from build123d import *

# Parameters (mm, degrees)
SKETCH1_W           = 100
SKETCH1_H           = 100
SKETCH1_R           = 0.75
BOSS_EXTRUDE1_DEPTH = 10
SKETCH2_W           = 110
SKETCH2_H           = 110
SKETCH2_W_2         = 100
SKETCH2_H_2         = 100
BOSS_EXTRUDE3_DEPTH = 5
FILLET2_R           = 2


with BuildPart() as part:
    # Sketch1 → Boss-Extrude1 (new body)
    with BuildSketch(Plane(origin=(0, 0, 0), x_dir=(1, 0, 0), z_dir=(0, 1, 0))):
        Rectangle(SKETCH1_W, SKETCH1_H)
        with Locations(Location((-25, 25, 0), (0, 0, 270))):
            Circle(SKETCH1_R, mode=Mode.SUBTRACT)
        with Locations(Location((25, -25, 0), (0, 0, 90))):
            Circle(SKETCH1_R, mode=Mode.SUBTRACT)
        with Locations(Location((25, 25, 0), (0, 0, 270))):
            Circle(SKETCH1_R, mode=Mode.SUBTRACT)
        with Locations(Location((-25, -25, 0), (0, 0, 90))):
            Circle(SKETCH1_R, mode=Mode.SUBTRACT)
    extrude(amount=BOSS_EXTRUDE1_DEPTH)

    # Sketch2 → Boss-Extrude3 (add)
    with BuildSketch(Plane(origin=(0, 10, 0), x_dir=(1, 0, 0), z_dir=(0, 1, 0))):
        Rectangle(SKETCH2_W, SKETCH2_H)
        Rectangle(SKETCH2_W_2, SKETCH2_H_2, mode=Mode.SUBTRACT)
    extrude(amount=-BOSS_EXTRUDE3_DEPTH)

    # Fillet2
    fillet2_edges = [part.edges().sort_by_distance(p)[0] for p in [
        (0, 5, -55),
        (-55, 7.5, -55),
        (55, 5, 0),
        (55, 7.5, -55),
        (0, 5, 55),
        (55, 7.5, 55),
        (-55, 5, 0),
        (-55, 7.5, 55),
        (0, 10, -55),
        (-55, 10, 0),
        (0, 10, 55),
        (55, 10, 0),
    ]]
    fillet(fillet2_edges, radius=FILLET2_R)


solid = part.part
Here's how the part is built. I have some questions about the finished solid (model axes, mm). A direction names the side the tool comes from. Give positions to 0.01 mm unless a question says otherwise; leave off trailing zeros. Write each loop counter-clockwise with the first axis right and the second up, starting at its lowest first coordinate (ties: lowest second). Pieces come first, ordered by that corner, then holes. Notation, with made-up numbers: (10, -33) -> (35, -33) arc R22 cw to (35, -2) -> close; hole circle Ø10 at (31, 55). An arc over 180 degrees is marked (long way). Use one line per item in the form item = value. Start each with the question number.
1. If I drill on L1, parallel to X at y = 4.5, z = -25; L2, parallel to X at y = 7, z = 25; L3, parallel to X at y = 4.25, z = 12, over which ranges is the centre line in solid material (lowest first)?
2. Will these pins go through, and if not, where does the flat tip stop? pin 1 Ø1.5 at (y, z) = (3.5, 2) entering from -X; pin 2 Ø2 at (x, z) = (37, 10) entering from -Y; pin 3 Ø0.9 at (x, z) = (-25, -25) entering from +Y; pin 4 Ø2.5 at (x, y) = (-17, 2.5) entering from -Z.
3. Imagine slicing it at C-C on x = -32. List the corners of the cut face in (y, z) for me, plus the area to 3 significant figures.
4. Imagine slicing it at B-B on y = 2. List the corners of the cut face in (x, z) for me.
5. Imagine slicing it at A-A on z = 16. List the corners of the cut face in (x, y) for me, plus the area to 3 significant figures.
6. On a 3-axis mill with a long thin cutter (end or side, diameter ignored), from which of +Z, -Z, +X, -X, +Y, -Y can I reach the whole of each face in a straight line? I mean faces 1 (the face through (50, 2, 1)), 2 (the face through (-1, 10, -1)), 3 (the face through (-1, 2, 50)), 4 (the face through (-50, 2, 1)), 5 (the face through (-1, 2, -50)). Say none if no direction works.
Entries:
q1.L1 = -50 to -25.75, -24.25 to 24.25, 25.75 to 50
q1.L2 = -55 to -25.75, -24.25 to 24.25, 25.75 to 55
q1.L3 = -50 to 50
q2.pin_1 = -50
q2.pin_2 = 0
q2.pin_3 = through
q2.pin_4 = -50
q3.outline = (0, -50) -> (5, -50) -> (5, -53) arc R2 ccw to (7, -55) -> (8, -55) arc R2 ccw to (10, -53) -> (10, 53) arc R2 ccw to (8, 55) -> (7, 55) arc R2 ccw to (5, 53) -> (5, 50) -> (0, 50) -> close
q3.area = 1,050 mm²
q4.outline = (-50, -50) -> (50, -50) -> (50, 50) -> (-50, 50) -> close; hole circle Ø1.5 at (-25, -25); hole circle Ø1.5 at (-25, 25); hole circle Ø1.5 at (25, -25); hole circle Ø1.5 at (25, 25)
q5.outline = (-55, 7) arc R2 ccw to (-53, 5) -> (-50, 5) -> (-50, 0) -> (50, 0) -> (50, 5) -> (53, 5) arc R2 ccw to (55, 7) -> (55, 8) arc R2 ccw to (53, 10) -> (-53, 10) arc R2 ccw to (-55, 8) -> close
q5.area = 1,050 mm²
q6.face_1 = +Z, -Z, +X, -Y
q6.face_2 = +Z, -Z, +X, -X, +Y
q6.face_3 = +Z, +X, -X, -Y
q6.face_4 = +Z, -Z, -X, -Y
q6.face_5 = -Z, +X, -X, -Y
